The listing builds one solid part. Answer for the finished solid, in the listing's coordinates (mm). Face numbers are marked on the shaded views. A direction names the side the tool comes from. Round coordinates to 2 decimals unless told otherwise and drop trailing zeros. Loops run counter-clockwise (first coordinate to the right, second up) from the corner with the lowest first, then second, coordinate; pieces in that order, holes last. Notation, with made-up numbers: M -38.5,22.5 L -6.5,22.5 A25 cw -6.5,46.5 Z; hole C 51,-29 d11. An arc over 180 degrees is marked long. Put each result on its own line as item: value. Start each with the question number.
(1) Which of the six approach directions +Z, -Z, +X, -X, +Y, -Y give full straight-line access (tool end or side, diameter ignored) to the marked faces 5 and 6?
(2) Section D-D, the plane y = -30.5 is taken. Determine the outline of the cut face in (x, z).
(3) Straight lines are drawn through the part: line 1 (X direction, y = 26, z = 14); line 2 (Z direction, x = 33, y = 0); line 3 (Y direction, x = -9, z = 4.5). For each, find the intervals that lie inside material, in ascending order.
(4) Section A-A, the plane z = 48 is taken. Determine the outline of the cut face in (x, y), then the cut area to 3 significant figures.
(5) Determine the mould class of the marked faces 1, 2, 3 and 4 for opening direction Y: released by +Y, released by -Y, zero draft, split by the parting line, or undercut.
(6) Section B-B, the plane x = 0 is taken. Determine the outline of the cut face in (y, z), then the cut area to 3 significant figures.
(7) Section C-C, the plane y = 0 is taken. Determine the outline of the cut face in (x, z).
(8) A flat-ended cylindrical pin translates along its axis: P1, Ø9, axis at x = 0, y = -32.14, coming from the +Z side. Find the tip coordinate at first contact, or state that the pin passes through.
```python
from build123d import *

# Parameters (mm, degrees)
SKETCH_W        = 80
SKETCH_H        = 108
PAD_DEPTH       = 3
SKETCH001_W     = 80
SKETCH001_H     = 108
SKETCH001_W_2   = 70
SKETCH001_H_2   = 98
PAD001_DEPTH    = 50
SKETCH002_R     = 4
POCKET_DEPTH    = 5
SKETCH004_R     = 1.75
POCKET002_DEPTH = 125
SKETCH003_R     = 1.75
POCKET003_DEPTH = 105


with BuildPart() as part:
    # Sketch → Pad (new body)
    with BuildSketch(Plane.XY):
        with Locations((-5, 0)):
            Rectangle(SKETCH_W, SKETCH_H)
    extrude(amount=PAD_DEPTH)

    # Sketch001 → Pad001 (join)
    with BuildSketch(Plane.XY.offset(3)):
        with Locations((-5, 0)):
            Rectangle(SKETCH001_W, SKETCH001_H)
        with Locations((-5, 0)):
            Rectangle(SKETCH001_W_2, SKETCH001_H_2, mode=Mode.SUBTRACT)
    extrude(amount=PAD001_DEPTH)

    # Sketch002 → Pocket (cut)
    with BuildSketch(Plane.XY):
        with Locations((0, -32.139076)):
            Circle(SKETCH002_R)
    extrude(amount=POCKET_DEPTH, mode=Mode.SUBTRACT)

    # Sketch004 → Pocket002 (cut, symmetric)
    with BuildSketch(Plane.XZ.offset(52)):
        with Locations((-5, 48)):
            Circle(SKETCH004_R)
    extrude(amount=POCKET002_DEPTH, both=True, mode=Mode.SUBTRACT)

    # Sketch003 → Pocket003 (cut)
    with BuildSketch(Plane.YZ.offset(46.5)):
        with Locations((0, 48)):
            Circle(SKETCH003_R)
    extrude(amount=-POCKET003_DEPTH, mode=Mode.SUBTRACT)


solid = part.part
```
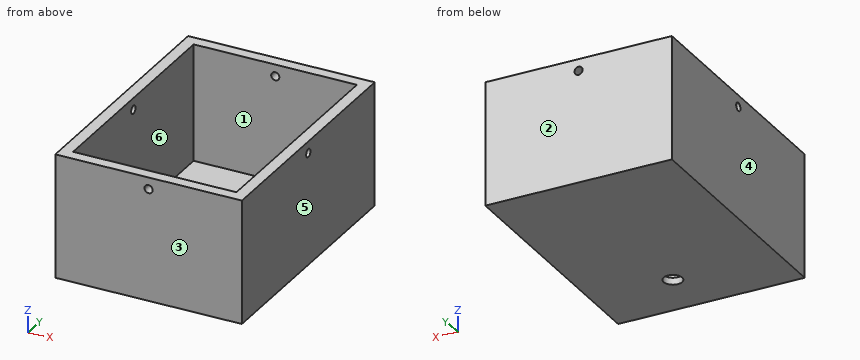
Recorded:
1. face 5: +Z, -Z, +X, +Y, -Y
1. face 6: +Z
2. outline: M -45,0 L -3.65,0 L -3.65,3 L -40,3 L -40,53 L -45,53 Z; M 3.65,0 L 35,0 L 35,53 L 30,53 L 30,3 L 3.65,3 Z
3. line 1: x = -45 to -40, 30 to 35
3. line 2: z = 0 to 46.25, 49.75 to 53
3. line 3: y = -54 to -49, 49 to 54
4. outline: M -45,-54 L -6.75,-54 L -6.75,-49 L -40,-49 L -40,-1.75 L -45,-1.75 Z; M -45,1.75 L -40,1.75 L -40,49 L -6.75,49 L -6.75,54 L -45,54 Z; M -3.25,-54 L 35,-54 L 35,-1.75 L 30,-1.75 L 30,-49 L -3.25,-49 Z; M -3.25,49 L 30,49 L 30,1.75 L 35,1.75 L 35,54 L -3.25,54 Z
4. area: 1,710 mm²
5. face 1: undercut
5. face 2: released by +Y
5. face 3: released by -Y
5. face 4: zero draft
6. outline: M -54,0 L -36.14,0 L -36.14,3 L -49,3 L -49,53 L -54,53 Z; M -28.14,0 L 54,0 L 54,53 L 49,53 L 49,3 L -28.14,3 Z
6. area: 800 mm²
7. outline: M -45,0 L 35,0 L 35,46.25 L 30,46.25 L 30,3 L -40,3 L -40,46.25 L -45,46.25 Z; M -45,49.75 L -40,49.75 L -40,53 L -45,53 Z; M 30,49.75 L 35,49.75 L 35,53 L 30,53 Z
8. P1: stops at z = 3
